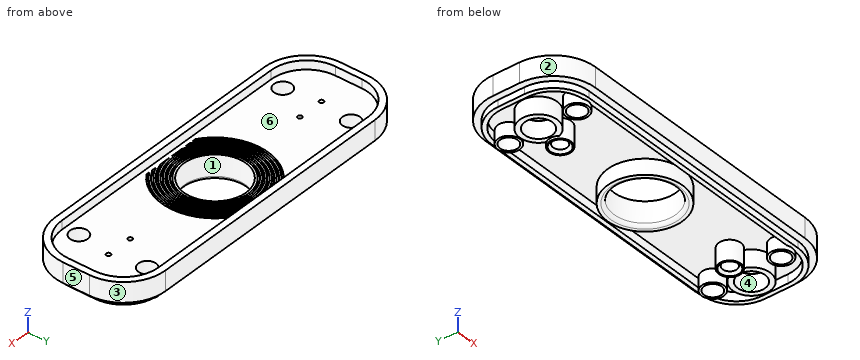
from build123d import *

# Parameters (mm, degrees)
BOSS_EXTRUDE1_DEPTH      = 1
BOSS_EXTRUDE2_DEPTH      = 3
BOSS_EXTRUDE2_DEPTH_BACK = 1.5
BOSS_EXTRUDE3_DEPTH      = 2
SKETCH3_R                = 7
SKETCH3_R_2              = 2
SKETCH3_R_3              = 0.5
CUT_EXTRUDE1_DEPTH       = 41.675545479
SKETCH4_R                = 8.5
SKETCH4_R_2              = 7
BOSS_EXTRUDE4_DEPTH      = 3.5
SKETCH5_R                = 4.25
SKETCH5_R_2              = 3.1
BOSS_EXTRUDE5_DEPTH      = 3.9
SKETCH6_R                = 2.5
SKETCH6_R_2              = 1.6
BOSS_EXTRUDE6_DEPTH      = 4.5
SKETCH7_R                = 2.5
SKETCH7_R_2              = 2
BOSS_EXTRUDE7_DEPTH      = 3
FILLET1_R                = 0.75
CHAMFER1_SIZE            = 0.75
CHAMFER2_SIZE            = 0.6
SKETCH8_R                = 9.583333337
SKETCH8_R_2              = 9.16666667
SKETCH8_R_3              = 8.750000003
SKETCH8_R_4              = 8.333333337
SKETCH8_R_5              = 7.91666667
SKETCH8_R_6              = 7.5
CUT_EXTRUDE6_DEPTH       = 0.5


with BuildPart() as part:
    # Sketch1 → Boss-Extrude1 (new, symmetric)
    with BuildSketch(Plane.XY):
        with BuildLine():
            Line((-29, 11), (29, 11))
            ThreePointArc((29, 11), (34.656854249, 8.656854249), (37, 3))
            Line((37, 3), (37, -3))
            ThreePointArc((37, -3), (34.656854249, -8.656854249), (29, -11))
            Line((29, -11), (-29, -11))
            ThreePointArc((-29, -11), (-34.656854249, -8.656854249), (-37, -3))
            Line((-37, -3), (-37, 3))
            ThreePointArc((-37, 3), (-34.656854249, 8.656854249), (-29, 11))
        make_face()
    extrude(amount=BOSS_EXTRUDE1_DEPTH, both=True)

    # Sketch1_4 → Boss-Extrude2 (add, two sides)
    with BuildSketch(Plane.XY) as boss_extrude2_sk:
        with BuildLine():
            Line((-29, 12.5), (29, 12.5))
            ThreePointArc((29, 12.5), (35.717514421, 9.717514421), (38.5, 3))
            Line((38.5, 3), (38.5, -3))
            ThreePointArc((38.5, -3), (35.717514421, -9.717514421), (29, -12.5))
            Line((29, -12.5), (-29, -12.5))
            ThreePointArc((-29, -12.5), (-35.717514421, -9.717514421), (-38.5, -3))
            Line((-38.5, -3), (-38.5, 3))
            ThreePointArc((-38.5, 3), (-35.717514421, 9.717514421), (-29, 12.5))
        make_face()
        with BuildLine():
            Line((-29, 11), (29, 11))
            ThreePointArc((29, 11), (34.656854249, 8.656854249), (37, 3))
            Line((37, 3), (37, -3))
            ThreePointArc((37, -3), (34.656854249, -8.656854249), (29, -11))
            Line((29, -11), (-29, -11))
            ThreePointArc((-29, -11), (-34.656854249, -8.656854249), (-37, -3))
            Line((-37, -3), (-37, 3))
            ThreePointArc((-37, 3), (-34.656854249, 8.656854249), (-29, 11))
        make_face(mode=Mode.SUBTRACT)
    extrude(amount=BOSS_EXTRUDE2_DEPTH)
    extrude(boss_extrude2_sk.sketch, amount=-BOSS_EXTRUDE2_DEPTH_BACK)

    # Sketch2 → Boss-Extrude3 (add)
    with BuildSketch(Plane(origin=(0, 0, -1), x_dir=(-1, 0, 0), z_dir=(0, 0, -1))):
        with BuildLine():
            Line((29, 11), (-29, 11))
            ThreePointArc((-29, 11), (-34.656854249, 8.656854249), (-37, 3))
            Line((-37, 3), (-37, -3))
            ThreePointArc((-37, -3), (-34.656854249, -8.656854249), (-29, -11))
            Line((-29, -11), (29, -11))
            ThreePointArc((29, -11), (34.656854249, -8.656854249), (37, -3))
            Line((37, -3), (37, 3))
            ThreePointArc((37, 3), (34.656854249, 8.656854249), (29, 11))
        make_face()
        with BuildLine():
            Line((29, 10), (-29, 10))
            ThreePointArc((-29, 10), (-33.949747468, 7.949747468), (-36, 3))
            Line((-36, 3), (-36, -3))
            ThreePointArc((-36, -3), (-33.949747468, -7.949747468), (-29, -10))
            Line((-29, -10), (29, -10))
            ThreePointArc((29, -10), (33.949747468, -7.949747468), (36, -3))
            Line((36, -3), (36, 3))
            ThreePointArc((36, 3), (33.949747468, 7.949747468), (29, 10))
        make_face(mode=Mode.SUBTRACT)
    extrude(amount=BOSS_EXTRUDE3_DEPTH)

    # Sketch3 → Cut-Extrude1 (cut, through all)
    with BuildSketch(Plane.XY.offset(1)):
        Circle(SKETCH3_R)
        with Locations((-28.25, 7.75)):
            Circle(SKETCH3_R_2)
        with Locations((28.25, 7.75)):
            Circle(SKETCH3_R_2)
        with Locations((28.25, -7.75)):
            Circle(SKETCH3_R_2)
        with Locations((-28.25, -7.75)):
            Circle(SKETCH3_R_2)
        with Locations((-29.5, 0)):
            Circle(SKETCH3_R_3)
        with Locations((29.5, 0)):
            Circle(SKETCH3_R_3)
        with Locations((23.5, 0)):
            Circle(SKETCH3_R_3)
        with Locations((-23.5, 0)):
            Circle(SKETCH3_R_3)
    extrude(amount=-CUT_EXTRUDE1_DEPTH, mode=Mode.SUBTRACT)

    # Sketch4 → Boss-Extrude4 (add)
    with BuildSketch(Plane(origin=(0, 0, -1), x_dir=(-1, 0, 0), z_dir=(0, 0, -1))):
        with Locations(Location((0, 0, 0), (0, 0, 180))):
            Circle(SKETCH4_R)
        with Locations(Location((0, 0, 0), (0, 0, 180))):
            Circle(SKETCH4_R_2, mode=Mode.SUBTRACT)
    extrude(amount=BOSS_EXTRUDE4_DEPTH)

    # Sketch5 → Boss-Extrude5 (add)
    with BuildSketch(Plane(origin=(0, 0, -1), x_dir=(-1, 0, 0), z_dir=(0, 0, -1))):
        with Locations(Location((29.5, 0, 0), (0, 0, 180))):
            Circle(SKETCH5_R)
        with Locations((29.5, 0)):
            Circle(SKETCH5_R_2, mode=Mode.SUBTRACT)
        with Locations(Location((-29.5, 0, 0), (0, 0, 180))):
            Circle(SKETCH5_R)
        with Locations((-29.5, 0)):
            Circle(SKETCH5_R_2, mode=Mode.SUBTRACT)
    extrude(amount=BOSS_EXTRUDE5_DEPTH)

    # Sketch6 → Boss-Extrude6 (add)
    with BuildSketch(Plane(origin=(0, 0, -1), x_dir=(-1, 0, 0), z_dir=(0, 0, -1))):
        with Locations(Location((23.5, 0, 0), (0, 0, 323.731147776))):
            Circle(SKETCH6_R)
        with Locations((23.5, 0)):
            Circle(SKETCH6_R_2, mode=Mode.SUBTRACT)
        with Locations(Location((-23.5, 0, 0), (0, 0, 216.268852224))):
            Circle(SKETCH6_R)
        with Locations((-23.5, 0)):
            Circle(SKETCH6_R_2, mode=Mode.SUBTRACT)
    extrude(amount=BOSS_EXTRUDE6_DEPTH)

    # Sketch7 → Boss-Extrude7 (add)
    with BuildSketch(Plane(origin=(0, 0, -1), x_dir=(-1, 0, 0), z_dir=(0, 0, -1))):
        with Locations(Location((-28.25, 7.75, 0), (0, 0, 116.320774831))):
            Circle(SKETCH7_R)
        with Locations(Location((-28.25, 7.75, 0), (0, 0, 180))):
            Circle(SKETCH7_R_2, mode=Mode.SUBTRACT)
        with Locations(Location((-28.25, -7.75, 0), (0, 0, 243.679225169))):
            Circle(SKETCH7_R)
        with Locations(Location((-28.25, -7.75, 0), (0, 0, 180))):
            Circle(SKETCH7_R_2, mode=Mode.SUBTRACT)
        with Locations(Location((28.25, 7.75, 0), (0, 0, 115.841932763))):
            Circle(SKETCH7_R)
        with Locations(Location((28.25, 7.75, 0), (0, 0, 180))):
            Circle(SKETCH7_R_2, mode=Mode.SUBTRACT)
        with Locations(Location((28.25, -7.75, 0), (0, 0, 244.158067237))):
            Circle(SKETCH7_R)
        with Locations(Location((28.25, -7.75, 0), (0, 0, 180))):
            Circle(SKETCH7_R_2, mode=Mode.SUBTRACT)
    extrude(amount=BOSS_EXTRUDE7_DEPTH)

    # Fillet1
    fillet1_edges = [part.edges().sort_by_distance(p)[0] for p in [
        (-7, 0, -4.5),
    ]]
    fillet(fillet1_edges, radius=FILLET1_R)

    # Chamfer1
    chamfer1_edges = [part.edges().sort_by_distance(p)[0] for p in [
        (-24, 0, -1),
        (23, 0, -1),
        (29, 0, -1),
        (-30, 0, -1),
    ]]
    chamfer(chamfer1_edges, length=CHAMFER1_SIZE)

    # Chamfer2
    chamfer2_edges = [part.edges().sort_by_distance(p)[0] for p in [
        (-21.9, 0, -5.5),
        (25.1, 0, -5.5),
    ]]
    chamfer(chamfer2_edges, length=CHAMFER2_SIZE)

    # Sketch8 → Cut-Extrude6 (cut)
    with BuildSketch(Plane.XY.offset(1)):
        Circle(SKETCH8_R)
        Circle(SKETCH8_R_2, mode=Mode.SUBTRACT)
        Circle(SKETCH8_R_3)
        Circle(SKETCH8_R_4, mode=Mode.SUBTRACT)
        Circle(SKETCH8_R_5)
        Circle(SKETCH8_R_6, mode=Mode.SUBTRACT)
        with BuildLine():
            Line((-0.258220535, 10), (-2.928549141, 10))
            ThreePointArc((-2.928549141, 10), (-10.420000003, 0), (-2.928549141, -10))
            Line((-2.928549141, -10), (-0.258220535, -10))
            ThreePointArc((-0.258220535, -10), (-10.003333337, 0), (-0.258220535, 10))
        make_face()
        with BuildLine():
            Line((-4.175325678, 10), (-5.161154056, 10))
            ThreePointArc((-5.161154056, 10), (-11.253333337, 0), (-5.161154056, -10))
            Line((-5.161154056, -10), (-4.175325678, -10))
            ThreePointArc((-4.175325678, -10), (-10.83666667, 0), (-4.175325678, 10))
        make_face()
        with BuildLine():
            Line((-6.015721077, 10), (-6.788778328, 10))
            ThreePointArc((-6.788778328, 10), (-12.08666667, 0), (-6.788778328, -10))
            Line((-6.788778328, -10), (-6.015721077, -10))
            ThreePointArc((-6.015721077, -10), (-11.670000003, 0), (-6.015721077, 10))
        make_face()
        with BuildLine():
            Line((2.928549141, 10), (0.258220535, 10))
            ThreePointArc((0.258220535, 10), (7.164137908, 6.981533204), (10.003333337, 0))
            ThreePointArc((10.003333337, 0), (7.164137908, -6.981533204), (0.258220535, -10))
            Line((0.258220535, -10), (2.928549141, -10))
            ThreePointArc((2.928549141, -10), (10.420000003, 0), (2.928549141, 10))
        make_face()
        with BuildLine():
            Line((5.161154056, 10), (4.175325678, 10))
            ThreePointArc((4.175325678, 10), (10.83666667, 0), (4.175325678, -10))
            Line((4.175325678, -10), (5.161154056, -10))
            ThreePointArc((5.161154056, -10), (11.253333337, 0), (5.161154056, 10))
        make_face()
        with BuildLine():
            Line((6.788778328, 10), (6.015721077, 10))
            ThreePointArc((6.015721077, 10), (11.670000003, 0), (6.015721077, -10))
            Line((6.015721077, -10), (6.788778328, -10))
            ThreePointArc((6.788778328, -10), (12.08666667, 0), (6.788778328, 10))
        make_face()
    extrude(amount=-CUT_EXTRUDE6_DEPTH, mode=Mode.SUBTRACT)


solid = part.part
Read the model definition and answer for the solid it produces. Units are mm, in the model's axes. Face numbers are marked on the shaded views. A direction names the side the tool comes from. Coordinates: 2 decimals unless noted, no trailing zeros. Order: outer loops, then holes, each group sorted by start corner. A loop starts at its lowest first (then second) coordinate and runs counter-clockwise, first axis right, second up. Notation, with made-up numbers: (42.5, 54) - (88.5, 54) arc R12 cw to (88.5, 70) - close; hole circle Ø7 at (84.5, 6.5). An arc over 180 degrees is marked (long way). Use one line per item in the form item = value.
(1) For a pull along Y with two mould halves and no side action, classify the marked faces 1, 2 and 3 as pulls with the +Y half, pulls with the -Y half, needs draft (parallel to the pull), parting line crosses it, or undercut.
Computed values:
face_1 = undercut
face_2 = pulls with the -Y half
face_3 = pulls with the +Y half
(2) Which of the six approach directions +Z, -Z, +X, -X, +Y, -Y give full straight-line access (tool end or side, diameter ignored) to the marked faces 4, 5 and 6?
Computed values:
face_4 = -Z
face_5 = +Z, -Z, +X, +Y, -Y
face_6 = +Z
(3) Straight lines are drawn through the part: L1, parallel to Y at x = -23.5, z = -2.05; L2, parallel to Y at x = 29.5, z = -4.05; L3, parallel to Y at x = 28.25, z = -0.85. For each, find the intervals that lie inside material, in ascending order.
Computed values:
L1 = -11 to -10, -2.5 to -1.6, 1.6 to 2.5, 10 to 11
L2 = -4.25 to -3.1, 3.1 to 4.25
L3 = -12.5 to -9.75, -5.75 to 5.75, 9.75 to 12.5
(4) Section B-B, the plane x = 15 is taken. Give the vertices of the cut face in (y, z), then the cut area to 3 significant figures.
Computed values:
outline = (-12.5, -1.5) - (-11, -1.5) - (-11, -3) - (-10, -3) - (-10, -1) - (10, -1) - (10, -3) - (11, -3) - (11, -1.5) - (12.5, -1.5) - (12.5, 3) - (11, 3) - (11, 1) - (-11, 1) - (-11, 3) - (-12.5, 3) - close
area = 61.5 mm²
(5) Given pin 1 Ø11 at (x, y) = (13, 3.5) entering from +Z; pin 2 Ø1.5 at (y, z) = (1, -2.5) entering from +X; pin 3 Ø1.5 at (x, y) = (-27.5, 8) entering from -Z (3 decimals); pin 4 Ø3.5 at (x, y) = (23.5, 0) entering from -Z, each flat-ended and moving along its own axis, determine where each tip first touches the part or whether it passes through.
Computed values:
pin_1 = 1
pin_2 = 37
pin_3 = through
pin_4 = -5.05
(6) Section A-A, the plane z = 2 is taken. Give the vertices of the cut face in (x, y).
Computed values:
outline = (-38.5, -3) arc R9.5 ccw to (-29, -12.5) - (29, -12.5) arc R9.5 ccw to (38.5, -3) - (38.5, 3) arc R9.5 ccw to (29, 12.5) - (-29, 12.5) arc R9.5 ccw to (-38.5, 3) - close; hole (-37, -3) arc R8 ccw to (-29, -11) - (29, -11) arc R8 ccw to (37, -3) - (37, 3) arc R8 ccw to (29, 11) - (-29, 11) arc R8 ccw to (-37, 3) - close
